from build123d import *

# Parameters (mm, degrees)
SKETCH_R        = 13
PAD_DEPTH       = 16
SKETCH001_R     = 14
PAD001_DEPTH    = 1
SKETCH002_R     = 14
PAD002_DEPTH    = 1
SKETCH003_R     = 8
POCKET_DEPTH    = 18.001
SKETCH004_W     = 70
SKETCH004_H     = 1
POCKET001_DEPTH = 17.9
CHAMFER_SIZE    = 0.8


with BuildPart() as part:
    # Sketch → Pad (new body)
    with BuildSketch(Plane.XY):
        Circle(SKETCH_R)
    extrude(amount=PAD_DEPTH)

    # Sketch001 → Pad001 (new body)
    with BuildSketch(Plane.XY.offset(16)):
        Circle(SKETCH001_R)
    extrude(amount=PAD001_DEPTH)

    # Sketch002 → Pad002 (new body)
    with BuildSketch(Plane(origin=(0, 0, 0), x_dir=(1, 0, 0), z_dir=(0, 0, -1))):
        Circle(SKETCH002_R)
    extrude(amount=PAD002_DEPTH)

    # Sketch003 → Pocket (cut, through all)
    with BuildSketch(Plane.XY.offset(17)):
        with Locations((3.5, 0)):
            Circle(SKETCH003_R)
    extrude(amount=-POCKET_DEPTH, mode=Mode.SUBTRACT)

    # Sketch004 → Pocket001 (cut)
    with BuildSketch(Plane(origin=(0, 0, -1), x_dir=(1, 0, 0), z_dir=(0, 0, -1))):
        Rectangle(SKETCH004_W, SKETCH004_H)
    extrude(amount=-POCKET001_DEPTH, mode=Mode.SUBTRACT)

    # Chamfer
    chamfer_edges = [part.edges().sort_by_distance(p)[0] for p in [
        (0, 14, 16),
        (0, -14, 16),
        (0, -14, 0),
        (0, 14, 0),
    ]]
    chamfer(chamfer_edges, length=CHAMFER_SIZE)


solid = part.part
The listing builds one solid part. Answer for the finished solid, in the listing's coordinates (mm). A direction names the side the tool comes from. Round coordinates to 2 decimals unless told otherwise and drop trailing zeros. Loops run counter-clockwise (first coordinate to the right, second up) from the corner with the lowest first, then second, coordinate; pieces in that order, holes last. Notation, with made-up numbers: M -16.5,75.25 L 21.5,75.25 A11 cw 21.5,85.25 Z; hole C -34.5,52.25 d8. An arc over 180 degrees is marked long. Write each question's results on one line, items separated by ' | '. Start each with the question number.
1) Find section A-A on z = 10.75. Write down the section's boundary in (x, y), plus the area to 3 significant figures.
2) Determine the mould class of faces 1 (the flat face through (12, -0.5, 8)), 2 (the conical face through (0.286, 13.325, 16.128)), 3 (the flat face through (-0.2, -7.3, -1)), 4 (the cylindrical face through (10.89, -3.06, 8.13)) for opening direction Y: pulls with the +Y half, pulls with the -Y half, needs draft (parallel to the pull), parting line crosses it, or undercut.
3) Straight lines are drawn through the part: probe 1 along Y at (x, z) = (8, 13); probe 2 along Y at (x, z) = (0, 10.5); probe 3 along X at (y, z) = (1, 12). For each, find the intervals that lie inside material, in ascending order.
4) Find section B-B on x = 0. Write down the section's boundary in (y, z), plus the area to 3 significant figures.
5) Each of these flat-tipped pins is pushed along its axis until it touches: pin 1 (14.5 mm diameter, centred on x = 3.5, y = 0, fed in from +Z); pin 2 (4 mm diameter, centred on y = -10, z = 11, fed in from -X); pin 3 (1 mm diameter, centred on y = -8, z = 8.5, fed in from +X); pin 4 (7.5 mm diameter, centred on x = -9.5, z = 12.5, fed in from +Y). Where does it stop, or does it pass through?
6) Which of the six approach directions +Z, -Z, +X, -X, +Y, -Y give full straight-line access (tool end or side, diameter ignored) to faces 5 (the flat face through (12, 0.5, 8)), 6 (the conical face through (-0.286, -13.325, 16.128)), 7 (the flat face through (-6, -3, 17)), 8 (the cylindrical face through (0, 13, 8))?
Final values:
1) outline: M -12.99,-0.5 A13 ccw 12.99,-0.5 L 11.48,-0.5 A8 cw -4.48,-0.5 Z; M -12.99,0.5 L -4.48,0.5 A8 cw 11.48,0.5 L 12.99,0.5 A13 ccw Z | area: 320 mm²
2) face 1: undercut | face 2: pulls with the +Y half | face 3: needs draft | face 4: undercut
3) probe 1: -10.25 to -6.61, 6.61 to 10.25 | probe 2: -13 to -7.19, 7.19 to 13 | probe 3: -12.96 to -4.44, 11.44 to 12.96
4) outline: M -14,-1 L -7.19,-1 L -7.19,17 L -14,17 L -14,16.8 L -13.2,16 L -13,16 L -13,0 L -13.2,0 L -14,-0.8 Z; M 7.19,-1 L 14,-1 L 14,-0.8 L 13.2,0 L 13,0 L 13,16 L 13.2,16 L 14,16.8 L 14,17 L 7.19,17 Z | area: 212 mm²
5) pin 1: through | pin 2: x = -10.25 | pin 3: x = 10.62 | pin 4: y = 11.66
6) face 5: -Z, +X, -X | face 6: -Y | face 7: +Z, +X, -X, +Y, -Y | face 8: +Y
